```python
from build123d import *

# Parameters (mm, degrees)
SKETCH_1_W          = 90
SKETCH_1_H          = 51
SKETCH_1_R          = 1.6
SKETCH_1_W_2        = 23
SKETCH_1_H_2        = 10.4
SKETCH_1_H_3        = 14.4
SKETCH_1_W_3        = 5.3
SKETCH_1_H_4        = 12.9
EXTRUDE_1_DEPTH     = 10
FILLET_1_R          = 2
EXTRUDE_START       = 5
SKETCH_2_R          = 3
SKETCH_2_R_2        = 1.6
EXTRUDE_2_DEPTH     = 5
FILLET_2_R          = 3
CUT_EXTRUDE_START   = -2.2
SKETCH_3_R          = 3
CUT_EXTRUDE_1_DEPTH = 2.2


with BuildPart() as part:
    # ｽｹｯﾁ1 → ﾎﾞｽ - 押し出し1 (new body)
    with BuildSketch(Plane(origin=(0, 0, 0), x_dir=(1, 0, 0), z_dir=(0, 1, 0))):
        with Locations((45, 25.5)):
            Rectangle(SKETCH_1_W, SKETCH_1_H)
        with Locations(Location((5, 46, 0), (0, 0, 270))):
            Circle(SKETCH_1_R, mode=Mode.SUBTRACT)
        with Locations(Location((85, 46, 0), (0, 0, 90))):
            Circle(SKETCH_1_R, mode=Mode.SUBTRACT)
        with Locations(Location((85, 5, 0), (0, 0, 270))):
            Circle(SKETCH_1_R, mode=Mode.SUBTRACT)
        with Locations(Location((5, 5, 0), (0, 0, 90))):
            Circle(SKETCH_1_R, mode=Mode.SUBTRACT)
        with Locations((26.1, 38.95)):
            Rectangle(SKETCH_1_W_2, SKETCH_1_H_2, mode=Mode.SUBTRACT)
        with Locations((63.65, 38.95)):
            Rectangle(SKETCH_1_W_2, SKETCH_1_H_3, mode=Mode.SUBTRACT)
        with Locations((27.3, 14.65)):
            Rectangle(SKETCH_1_W_3, SKETCH_1_H_4, mode=Mode.SUBTRACT)
        with Locations((62.7, 14.65)):
            Rectangle(SKETCH_1_W_3, SKETCH_1_H_4, mode=Mode.SUBTRACT)
    extrude(amount=EXTRUDE_1_DEPTH)

    # ﾌｨﾚｯﾄ1
    fillet_1_edges = [part.edges().sort_by_distance(p)[0] for p in [
        (60.05, 5, -21.1),
        (60.05, 5, -8.2),
        (65.35, 5, -8.2),
        (65.35, 5, -21.1),
        (29.95, 5, -21.1),
        (24.65, 5, -21.1),
        (24.65, 5, -8.2),
        (29.95, 5, -8.2),
    ]]
    fillet(fillet_1_edges, radius=FILLET_1_R)

    # ｽｹｯﾁ2 → ﾎﾞｽ - 押し出し2 (add)
    # profile 1 of 4: a face of its own
    with BuildSketch(Plane.XZ.offset(EXTRUDE_START)):
        with Locations(Location((5, -5, 0), (0, 0, 270))):
            Circle(SKETCH_2_R)
        with Locations(Location((5, -5, 0), (0, 0, 270))):
            Circle(SKETCH_2_R_2, mode=Mode.SUBTRACT)
    # profile 2 of 4: a face of its own
    with BuildSketch(Plane.XZ.offset(EXTRUDE_START)):
        with Locations(Location((85, -5, 0), (0, 0, 90))):
            Circle(SKETCH_2_R)
        with Locations(Location((85, -5, 0), (0, 0, 90))):
            Circle(SKETCH_2_R_2, mode=Mode.SUBTRACT)
    # profile 3 of 4: a face of its own
    with BuildSketch(Plane.XZ.offset(EXTRUDE_START)):
        with Locations(Location((85, -46, 0), (0, 0, 270))):
            Circle(SKETCH_2_R)
        with Locations(Location((85, -46, 0), (0, 0, 270))):
            Circle(SKETCH_2_R_2, mode=Mode.SUBTRACT)
    # profile 4 of 4: a face of its own
    with BuildSketch(Plane.XZ.offset(EXTRUDE_START)):
        with Locations(Location((5, -46, 0), (0, 0, 90))):
            Circle(SKETCH_2_R)
        with Locations(Location((5, -46, 0), (0, 0, 90))):
            Circle(SKETCH_2_R_2, mode=Mode.SUBTRACT)
    extrude(amount=-EXTRUDE_2_DEPTH)

    # ﾌｨﾚｯﾄ2
    fillet_2_edges = [part.edges().sort_by_distance(p)[0] for p in [
        (0, 5, -51),
        (90, 5, -51),
        (90, 5, 0),
        (0, 5, 0),
    ]]
    fillet(fillet_2_edges, radius=FILLET_2_R)

    # ｽｹｯﾁ3 → ｶｯﾄ - 押し出し1 (cut)
    with BuildSketch(Plane(origin=(0, 10, 0), x_dir=(1, 0, 0), z_dir=(0, 1, 0)).offset(CUT_EXTRUDE_START)):
        with Locations(Location((5, 46, 0), (0, 0, 270))):
            Circle(SKETCH_3_R)
        with Locations(Location((85, 46, 0), (0, 0, 90))):
            Circle(SKETCH_3_R)
        with Locations(Location((85, 5, 0), (0, 0, 270))):
            Circle(SKETCH_3_R)
        with Locations(Location((5, 5, 0), (0, 0, 90))):
            Circle(SKETCH_3_R)
    extrude(amount=CUT_EXTRUDE_1_DEPTH, mode=Mode.SUBTRACT)


solid = part.part
```
Design review of the part built by this model. Coordinates are the model's own, in mm. A direction names the side the tool comes from. Coordinates: 2 decimals unless noted, no trailing zeros. Order: outer loops, then holes, each group sorted by start corner. A loop starts at its lowest first (then second) coordinate and runs counter-clockwise, first axis right, second up.
1) Take a section at B-B, the plane x = 68.5. Give the boundary of the cut face in (y, z), and give its area (3 significant figures).
2) Take a section at C-C, the plane x = 85. Give the boundary of the cut face in (y, z).
3) Wall thickness on line 1 along X through (y, z) = (8.5, -5); line 2 along X through (y, z) = (9.35, -46); line 3 along X through (y, z) = (2.5, -46): over which ranges is each line inside the solid? List them lowest first.
4) Take a section at A-A, the plane z = -36.5. Give the boundary of the cut face in (x, y), and give its area (3 significant figures).
5) Take a section at D-D, the plane y = 1.5. State how many separate pieces and enclosed holes the cut face has, and give its area (3 significant figures).
6) Mouldability with a two-part tool opening along X and no side actions: class faces 1 (the cylindrical face through (0.86, 5.07, -0.9)), 2 (the cylindrical face through (89.1, 5.07, -50.14)), 3 (the flat face through (6.3, 7.8, -6.3)) as +X half, -X half, draft (parallel to the pull), parting line (faces both ways), or undercut.
7) Clearance check with flat-ended pins moving along their axes: pin 1 (2 mm diameter, centred on x = 20.5, z = -14.5, fed in from -Y); pin 2 (3.5 mm diameter, centred on x = 5, z = -5, fed in from +Y). State where each tip first meets the part, or that it passes through.
8) For faces 4 (the cylindrical face through (64.78, 5.07, -20.5)), 5 (the cylindrical face through (89.1, 5.07, -0.86)), 6 (the cylindrical face through (5, 9, -49)), list the 3-axis set-ups (+Z, -Z, +X, -X, +Y, -Y) from which the entire face can be reached by the end or side of a thin tool; tool diameter is ignored.
Returned:
1. outline: (0, -51) - (10, -51) - (10, -46.15) - (0, -46.15) - close; (0, -31.75) - (10, -31.75) - (10, 0) - (0, 0) - close
1. area: 366 mm2
2. outline: (-5, -49) - (0, -49) - (0, -51) - (10, -51) - (10, -49) - (7.8, -49) - (7.8, -47.6) - (-5, -47.6) - close; (-5, -44.4) - (7.8, -44.4) - (7.8, -43) - (10, -43) - (10, -8) - (7.8, -8) - (7.8, -6.6) - (-5, -6.6) - (-5, -8) - (0, -8) - (0, -43) - (-5, -43) - close; (-5, -3.4) - (7.8, -3.4) - (7.8, -2) - (10, -2) - (10, 0) - (0, 0) - (0, -2) - (-5, -2) - close
3. line 1: x = 0 to 2, 8 to 82, 88 to 90
3. line 2: x = 0 to 2, 8 to 52.15, 75.15 to 82, 88 to 90
3. line 3: x = 0 to 3.4, 6.6 to 52.15, 75.15 to 83.4, 86.6 to 90
4. outline: (0, 0) - (14.6, 0) - (14.6, 10) - (0, 10) - close; (37.6, 0) - (52.15, 0) - (52.15, 10) - (37.6, 10) - close; (75.15, 0) - (90, 0) - (90, 10) - (75.15, 10) - close
4. area: 440 mm2
5. separate pieces: 1
5. enclosed holes: 8
5. area: 3,850 mm2
6. face 1: -X half
6. face 2: +X half
6. face 3: undercut
7. pin 1: stops at y = 0
7. pin 2: stops at y = 7.8
8. face 4: +Y, -Y
8. face 5: +Z, +X, +Y, -Y
8. face 6: +Y
